Could you check a few things on this model? Use its own coordinates, in mm. Face numbers are marked on the shaded views. A direction names the side the tool comes from. Give positions to 0.01 mm unless a question says otherwise; leave off trailing zeros. Loops run counter-clockwise (first coordinate to the right, second up) from the corner with the lowest first, then second, coordinate; pieces in that order, holes last. Notation, with made-up numbers: M -38.75,52.5 L 1.25,52.5 A15 ccw 1.25,72.5 Z; hole C 11.25,66 d4. An arc over 180 degrees is marked long. Return JSON: item names as keys, results as strings. Group by question number.
1. If we section it at D-D (z = -51.5): Write out the boundary of the cut face in (x, y).
2. If we section it at B-B (x = 30.5): Write out the boundary of the cut face in (y, z), plus the area to 3 significant figures.
3. If we section it at C-C (z = -59.5): Write out the boundary of the cut face in (x, y), plus the area to 3 significant figures.
4. For pin 1 (1.5 mm diameter, centred on x = 53, y = 40.5, fed in from -Z); pin 2 (4 mm diameter, centred on x = 9.6, z = -21.5, fed in from +Y); pin 3 (1.2 mm diameter, centred on x = 42, y = 3, fed in from +Z); pin 4 (12 mm diameter, centred on x = 48.5, z = -15.5, fed in from +Y), each with a flat end and sliding along its axis, tell me the tip position at first contact or that it passes through.
5. If we section it at A-A (y = 32.5): Write out the boundary of the cut face in (x, z).
6. Please list where these lines run through material, in increasing order: line 1 (X direction, y = 3.25, z = -59.5); line 2 (X direction, y = 1.7, z = -21.5); line 3 (Y direction, x = 40, z = -19).
7. For the marked faces 1 and 2, which set-ups out of +Z, -Z, +X, -X, +Y, -Y let a thin tool reach every point of the face, with its end or its side?
```python
from build123d import *

# Parameters (mm, degrees)
SKETCH1_W           = 4
SKETCH1_H           = 52
SKETCH1_H_2         = 4
SKETCH1_W_2         = 62
BOSS_EXTRUDE1_DEPTH = 76
SKETCH2_R           = 2.5
CUT_EXTRUDE1_DEPTH  = 116.1868048
CUT_EXTRUDE2_DEPTH  = 116.1868048
FILLET1_R           = 5
FILLET2_R           = 2


with BuildPart() as part:
    # Sketch1 → Boss-Extrude1 (new body)
    with BuildSketch(Plane(origin=(0, 0, 0), x_dir=(0, 0, -1), z_dir=(1, 0, 0))):
        with Locations((2, 30)):
            Rectangle(SKETCH1_W, SKETCH1_H)
        with Locations((2, 2)):
            Rectangle(SKETCH1_W, SKETCH1_H_2)
        with Locations((35, 2)):
            Rectangle(SKETCH1_W_2, SKETCH1_H_2)
    extrude(amount=BOSS_EXTRUDE1_DEPTH)

    # Sketch2 → Cut-Extrude1 (cut, through all)
    with BuildSketch(Plane.XZ):
        with Locations(Location((9.6, -59.5, 0), (0, 0, 270))):
            Circle(SKETCH2_R)
        with Locations(Location((9.6, -21.5, 0), (0, 0, 270))):
            Circle(SKETCH2_R)
        with Locations(Location((23.6, -21.5, 0), (0, 0, 270))):
            Circle(SKETCH2_R)
        with Locations(Location((65.6, -21.5, 0), (0, 0, 270))):
            Circle(SKETCH2_R)
        with Locations(Location((65.6, -59.5, 0), (0, 0, 270))):
            Circle(SKETCH2_R)
        with Locations(Location((51.6, -59.5, 0), (0, 0, 270))):
            Circle(SKETCH2_R)
        with BuildLine():
            Line((54.5, -54), (21.5, -54))
            ThreePointArc((21.5, -54), (8, -40.5), (21.5, -27))
            Line((21.5, -27), (54.5, -27))
            ThreePointArc((54.5, -27), (68, -40.5), (54.5, -54))
        make_face()
    extrude(amount=-CUT_EXTRUDE1_DEPTH, mode=Mode.SUBTRACT)

    # Sketch3 → Cut-Extrude2 (cut, through all)
    with BuildSketch(Plane.XY):
        with BuildLine():
            Line((16, 48), (16, 15))
            ThreePointArc((16, 15), (13, 12), (10, 15))
            Line((10, 15), (10, 48))
            ThreePointArc((10, 48), (13, 51), (16, 48))
        make_face()
        with BuildLine():
            Line((60, 48), (60, 15))
            ThreePointArc((60, 15), (63, 12), (66, 15))
            Line((66, 15), (66, 48))
            ThreePointArc((66, 48), (63, 51), (60, 48))
        make_face()
    extrude(amount=-CUT_EXTRUDE2_DEPTH, mode=Mode.SUBTRACT)

    # Fillet1
    fillet1_edges = [part.edges().sort_by_distance(p)[0] for p in [
        (38, 0, 0),
        (76, 2, -66),
        (76, 56, -2),
        (0, 56, -2),
        (0, 2, -66),
    ]]
    fillet(fillet1_edges, radius=FILLET1_R)

    # Fillet2
    fillet2_edges = [part.edges().sort_by_distance(p)[0] for p in [
        (38, 4, -4),
    ]]
    fillet(fillet2_edges, radius=FILLET2_R)


solid = part.part
```
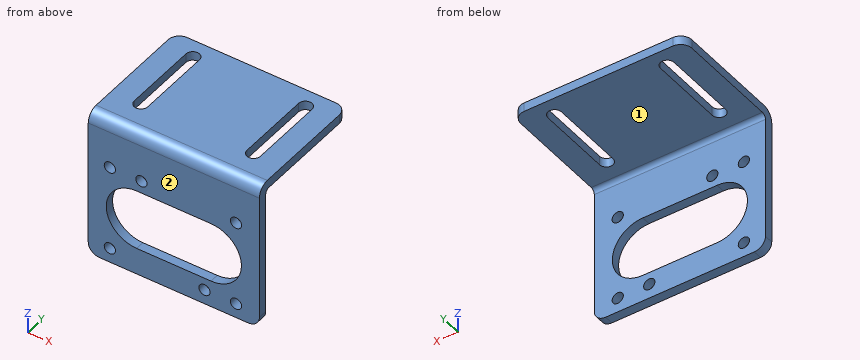
Answer:
{
 "1": {"outline": "M 0,0 L 13.67,0 L 13.67,4 L 0,4 Z; M 62.33,0 L 76,0 L 76,4 L 62.33,4 Z"},
 "2": {"outline": "M 0,-66 L 4,-66 L 4,-54 L 0,-54 Z; M 0,-27 L 4,-27 L 4,-6 A2 cw 6,-4 L 56,-4 L 56,0 L 5,0 A5 ccw 0,-5 Z", "area": "359 mm²"},
 "3": {"outline": "M 0,0 L 7.1,0 L 7.1,4 L 0,4 Z; M 12.1,0 L 49.1,0 L 49.1,4 L 12.1,4 Z; M 54.1,0 L 63.1,0 L 63.1,4 L 54.1,4 Z; M 68.1,0 L 76,0 L 76,4 L 68.1,4 Z", "area": "244 mm²"},
 "4": {"pin 1": "stops at z = -4", "pin 2": "passes through", "pin 3": "stops at z = -0.2", "pin 4": "stops at y = 4"},
 "5": {"outline": "M 0,-4 L 10,-4 L 10,0 L 0,0 Z; M 16,-4 L 60,-4 L 60,0 L 16,0 Z; M 66,-4 L 76,-4 L 76,0 L 66,0 Z"},
 "6": {"line 1": "x = 0 to 7.1, 12.1 to 49.1, 54.1 to 63.1, 68.1 to 76", "line 2": "x = 0 to 7.1, 12.1 to 21.1, 26.1 to 63.1, 68.1 to 76", "line 3": "y = 0 to 4"},
 "7": {"face 1": "-Z, +X, -X, +Y", "face 2": "+Z, -Z, +X, -X, -Y"}
}
